Can you work these out from the model? Positions are in its coordinate system, mm. Face numbers are marked on the shaded views. Round coordinates to 2 decimals unless told otherwise and drop trailing zeros. Order: outer loops, then holes, each group sorted by start corner. A loop starts at its lowest first (then second) coordinate and runs counter-clockwise, first axis right, second up. Notation, with made-up numbers: (13.25, 65.25) -> (43.25, 65.25) arc R25 cw to (43.25, 93.25) -> close; hole circle Ø5 at (-6.75, 33). An arc over 180 degrees is marked (long way). Use a Markdown table: item, result. Add a question column.
Q1. I need wall thicknesses on line 1 along X through (y, z) = (-7.8, -53); line 2 along Z through (x, y) = (71, -7.4); line 3 along Z through (x, y) = (64, -5.65). Which ranges of each line are inside material? Lowest first, please. Write a range as [from, to].
Q2. If we section it at B-B on x = 56: List the corners of the cut face in (y, z) for me.
Q3. If we section it at A-A on z = -53: List the corners of the cut face in (x, y) for me, plus the area to 3 significant figures.
Q4. If we section it at C-C on x = 64: List the corners of the cut face in (y, z) for me.
Q5. We'd pull the mould along Z, two halves only. Please class the marked faces 1, 2 and 3: +Z half, -Z half, draft (parallel to the pull), parting line (faces both ways), or undercut.
Q6. If we section it at D-D on x = 66.75: List the corners of the cut face in (y, z) for me.
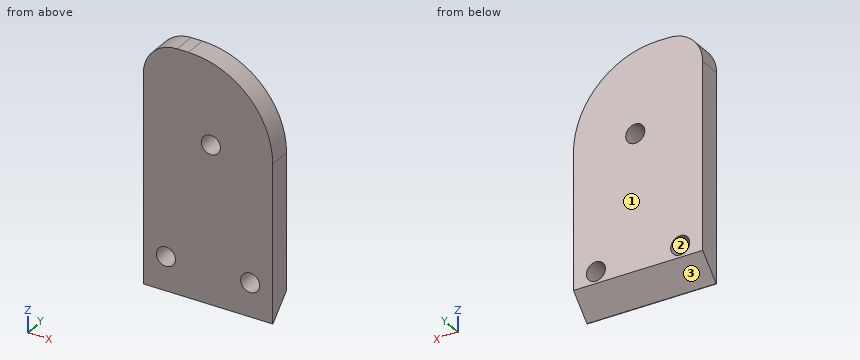
```python
from build123d import *

# Parameters (mm, degrees)
CYLINDER223_R          = 1.7
CYLINDER223_DEPTH      = 21
CYLINDER223_ROLL_ANGLE = 90
CYLINDER201_R          = 1.7
CYLINDER201_DEPTH      = 20
CYLINDER201_ROLL_ANGLE = 90
CYLINDER200_R          = 1.7
CYLINDER200_DEPTH      = 20
CYLINDER200_ROLL_ANGLE = 90
BOX001027045147_W      = 23
BOX001027045147_H      = 4
BOX001027045147_DEPTH  = 43
FILLET034_R            = 15
FILLET038_R            = 6
CHAMFER028_SIZE        = 3.9


with BuildPart() as bearing_fit_cylinder003:
    # Cylinder223 → Cylinder223 (new body)
    with BuildSketch(Plane.XY):
        Circle(CYLINDER223_R)
    extrude(amount=CYLINDER223_DEPTH)


with BuildPart() as bearing_fit_cylinder003_1:
    # Cylinder223 roll: moved
    add(bearing_fit_cylinder003.part.rotate(Axis((0, 0, 0), (1, 0, 0)), CYLINDER223_ROLL_ANGLE))


with BuildPart() as bearing_fit_cylinder003_2:
    # Cylinder223 placement: moved
    add(bearing_fit_cylinder003_1.part.moved(Location((64, 5, -31))))


with BuildPart() as cylinder245:
    # Cylinder201 → Cylinder201 (new body)
    with BuildSketch(Plane.XY):
        Circle(CYLINDER201_R)
    extrude(amount=CYLINDER201_DEPTH)


with BuildPart() as cylinder245_1:
    # Cylinder201 roll: moved
    add(cylinder245.part.rotate(Axis((0, 0, 0), (1, 0, 0)), CYLINDER201_ROLL_ANGLE))


with BuildPart() as cylinder245_2:
    # Cylinder201 placement: moved
    add(cylinder245_1.part.moved(Location((71, 8, -54))))


with BuildPart() as fusion112101:
    # Cylinder200 → Cylinder200 (new body)
    with BuildSketch(Plane.XY):
        Circle(CYLINDER200_R)
    extrude(amount=CYLINDER200_DEPTH)


with BuildPart() as fusion112101_1:
    # Cylinder200 roll: moved
    add(fusion112101.part.rotate(Axis((0, 0, 0), (1, 0, 0)), CYLINDER200_ROLL_ANGLE))


with BuildPart() as fusion112101_2:
    # Cylinder200 placement: moved
    add(fusion112101_1.part.moved(Location((56, 8, -54))))

    # Fusion112101: union Cylinder245
    add(cylinder245_2.part)


with BuildPart() as fusion112101_3:
    # Fusion112101 placement: moved
    add(fusion112101_2.part.moved(Location((0, 0, 1))))


with BuildPart() as chamfer028:
    # Box001027045147 → Box001027045147 (new body)
    with BuildSketch(Plane(origin=(52, -8.8, -59), x_dir=(1, 0, 0), z_dir=(0, 0, 1))):
        with Locations((11.5, 2)):
            Rectangle(BOX001027045147_W, BOX001027045147_H)
    extrude(amount=BOX001027045147_DEPTH)

    # Cut177: cut Fusion112101
    add(fusion112101_3.part, mode=Mode.SUBTRACT)

    # Cut201: cut bearing-fit-cylinder003
    add(bearing_fit_cylinder003_2.part, mode=Mode.SUBTRACT)

    # Fillet034
    fillet034_edges = [chamfer028.edges().sort_by_distance(p)[0] for p in [
        (75, -6.8, -16),
    ]]
    fillet(fillet034_edges, radius=FILLET034_R)

    # Fillet038
    fillet038_edges = [chamfer028.edges().sort_by_distance(p)[0] for p in [
        (52, -6.8, -16),
    ]]
    fillet(fillet038_edges, radius=FILLET038_R)

    # Chamfer028
    chamfer028_edges = [chamfer028.edges().sort_by_distance(p)[0] for p in [
        (63.5, -4.8, -59),
    ]]
    chamfer(chamfer028_edges, length=CHAMFER028_SIZE)


solid = chamfer028.part
```
Answer below:
| question | item | result |
|---|---|---|
| 1 | line 1 | [52, 54.3], [57.7, 69.3], [72.7, 75] |
| 1 | line 2 | [-57.7, -54.7], [-51.3, -20.8] |
| 1 | line 3 | [-55.95, -32.7], [-29.3, -16.54] |
| 2 | outline | (-8.8, -59) -> (-8.7, -59) -> (-4.8, -55.1) -> (-4.8, -54.7) -> (-8.8, -54.7) -> close; (-8.8, -51.3) -> (-4.8, -51.3) -> (-4.8, -16.34) -> (-8.8, -16.34) -> close |
| 3 | outline | (52, -8.8) -> (54.3, -8.8) -> (54.3, -4.8) -> (52, -4.8) -> close; (57.7, -8.8) -> (69.3, -8.8) -> (69.3, -4.8) -> (57.7, -4.8) -> close; (72.7, -8.8) -> (75, -8.8) -> (75, -4.8) -> (72.7, -4.8) -> close |
| 3 | area | 64.8 mm² |
| 4 | outline | (-8.8, -59) -> (-8.7, -59) -> (-4.8, -55.1) -> (-4.8, -32.7) -> (-8.8, -32.7) -> close; (-8.8, -29.3) -> (-4.8, -29.3) -> (-4.8, -16.54) -> (-8.8, -16.54) -> close |
| 5 | face 1 | draft |
| 5 | face 2 | undercut |
| 5 | face 3 | -Z half |
| 6 | outline | (-8.8, -59) -> (-8.7, -59) -> (-4.8, -55.1) -> (-4.8, -17.6) -> (-8.8, -17.6) -> close |
